For this review, take the finished solid that the model builds, in its own axes (mm). A direction names the side the tool comes from. Give positions to 0.01 mm unless a question says otherwise; leave off trailing zeros. Order: outer loops, then holes, each group sorted by start corner. A loop starts at its lowest first (then second) coordinate and runs counter-clockwise, first axis right, second up. Notation, with made-up numbers: M 8.25,86.25 L 35.25,86.25 A21 cw 35.25,98.25 Z; hole C -38.5,46.25 d1. An arc over 180 degrees is marked long. Use CSV: the item, a comma, the result in double quotes. Start each with the question number.
(1) Consider section D-D (x = 22.5). Write out the cut boundary in (y, z).
(2) Clearance check with flat-ended pins moving along their axes: P1, Ø9, axis at x = -1, z = -7.5, coming from the +Y side; P2, Ø1, axis at y = 4, z = 4.5, coming from the +X side; P3, Ø0.5, axis at x = 45.5, y = 3, coming from the +Z side; P4, Ø5, axis at x = 14.5, z = 2.5, coming from the +Y side. State where each tip first meets the part, or that it passes through.
(3) Consider section B-B (z = 33.5). Write out the cut boundary in (x, y).
(4) Tool access review of faces 1 (the face through (41.558, 2.768, 37.791)), 2 (the face through (-25.974, 3, 34)), 3 (the face through (-41.83, 0.99, -8.8)), 4 (the face through (-51, 2, 9.454)): name each direction out of +Z, -Z, +X, -X, +Y, -Y from which nothing blocks a thin tool from reaching the whole face with its end or side.
(5) Consider section A-A (x = 4). Write out the cut boundary in (y, z), and give its area (3 significant figures).
(6) Draft analysis for pull direction X (two halves, no side actions). For faces 5 (the face through (37, 4, 39)), 6 (the face through (14.226, 3, -3)), 7 (the face through (-42.463, 0.993, 41.416)), 8 (the face through (-48.627, 4, 15)), state which applies: pulls with the +X half, pulls with the -X half, needs draft (parallel to the pull), parting line crosses it, or undercut.
(7) Wall thickness on L1, parallel to Z at x = 2, y = 4.2; L2, parallel to X at y = 0.6, z = 41; L3, parallel to Z at x = -1, y = 1.1: over which ranges is each line inside the solid? List them lowest first. Write a range as from..to.
(8) Consider section C-C (z = 6.5). Write out the cut boundary in (x, y), and give its area (3 significant figures).
```python
from build123d import *

# Parameters (mm, degrees)
EXTRUDE_1_DEPTH     = 1.5
SKETCH_2_R          = 5
CUT_EXTRUDE_1_DEPTH = 0.5
SKETCH_11_R         = 2
SKETCH_11_W         = 12.230000074
SKETCH_11_H         = 11.974599949
EXTRUDE_5_DEPTH     = 2.539974634
SKETCH_13_R         = 2
SKETCH_13_W         = 4
SKETCH_13_H         = 10
TYPEC_2_DEPTH       = 5.7999746
LED_3_START         = -4.25
LED_3_DEPTH         = 2.75
LED_1_R             = 0.5
CUT_EXTRUDE_2_REACH = 75.864
SKETCH_15_R         = 2
EXTRUDE_START       = -4
SKETCH_16_R         = 4
SKETCH_16_R_2       = 1
EXTRUDE_4_DEPTH     = 2.5
LED_2_START         = -1.5
SKETCH_17_W         = 1
SKETCH_17_H         = 6
LED_2_DEPTH         = 0.5
SKETCH_18_W         = 40.2
SKETCH_18_H         = 3
EXTRUDE_2_DEPTH     = 3.5


with BuildPart() as part:
    # 草图1 → 凸台-拉伸1 (new body)
    with BuildSketch(Plane(origin=(0, 0, 0), x_dir=(1, 0, 0), z_dir=(0, 1, 0))):
        Polygon((-51.714401712, -9.454370264), (-55.976720775, -9.454370264), (-55.976720775, -21.428970213), (-51.714401712, -21.428970213), (-51.714401712, -47.841670238), (46.085598288, -47.841670238), (46.085598288, 16.958329762), (-51.714401712, 16.958329762), align=None)
    extrude(amount=EXTRUDE_1_DEPTH)

    # 草图2 → 防滑切除-拉伸1 (cut)
    with BuildSketch(Plane.XZ):
        with Locations(Location((-43.814401712, 39.941670238, 0), (0, 0, 270))):
            Circle(SKETCH_2_R)
        with Locations(Location((38.185598288, 39.941670238, 0), (0, 0, 90))):
            Circle(SKETCH_2_R)
        with Locations(Location((38.185598288, -9.058329762, 0), (0, 0, 90))):
            Circle(SKETCH_2_R)
        with Locations(Location((-43.814401712, -9.058329762, 0), (0, 0, 270))):
            Circle(SKETCH_2_R)
    extrude(amount=-CUT_EXTRUDE_1_DEPTH, mode=Mode.SUBTRACT)

    # 草图11 → 充电板档板凸台-拉伸5 (add)
    with BuildSketch(Plane.XZ):
        with Locations((-29.074401712, 29.928970213)):
            Circle(SKETCH_11_R)
        with Locations((-29.074401712, 0.954370264)):
            Circle(SKETCH_11_R)
        with Locations((-49.861720738, 15.441670239)):
            Rectangle(SKETCH_11_W, SKETCH_11_H)
    extrude(amount=-EXTRUDE_5_DEPTH)

    # 草图13 → TypeC支撑凸台-拉伸2 (add)
    with BuildSketch(Plane.XZ):
        with Locations(Location((-29.074401712, 29.928970213, 0), (0, 0, 90))):
            Circle(SKETCH_13_R)
        with Locations(Location((-29.074401712, 0.954370264, 0), (0, 0, 90))):
            Circle(SKETCH_13_R)
        with Locations((-46.626720701, 15.441670238)):
            Rectangle(SKETCH_13_W, SKETCH_13_H)
    extrude(amount=-TYPEC_2_DEPTH)

    # 草图14 → LED限位凸台-拉伸3 (add)
    with BuildSketch(Plane.XZ.offset(LED_3_START)):
        Polygon((45.085598288, 12.441670238), (45.085598288, 18.441670238), (46.085598288, 18.441670238), (46.085598288, 21.441670238), (42.085598288, 21.441670238), (42.085598288, 9.441670238), (46.085598288, 9.441670238), (46.085598288, 12.441670238), align=None)
    extrude(amount=LED_3_DEPTH)

    # LED限位圆角1
    led_1_edges = [part.edges().sort_by_distance(p)[0] for p in [
        (45.585598288, 4.25, 18.441670238),
        (45.585598288, 4.25, 12.441670238),
        (45.085598288, 4.25, 15.441670238),
        (-48.626720701, 5.7999746, 15.441670238),
    ]]
    fillet(led_1_edges, radius=LED_1_R)

    # 草图15 → 螺丝孔位切除-拉伸2 (cut, up to next)
    with BuildSketch(Plane.XZ, mode=Mode.PRIVATE) as cut_extrude_2_sk1:
        with Locations(Location((-43.814401712, -9.058329762, 0), (0, 0, 270))):
            Circle(SKETCH_15_R)
    cut_extrude_2_tool1 = extrude(cut_extrude_2_sk1.sketch, amount=-CUT_EXTRUDE_2_REACH, mode=Mode.PRIVATE) & part.part
    # 草图15 → 螺丝孔位切除-拉伸2 (cut, up to next)
    with BuildSketch(Plane.XZ, mode=Mode.PRIVATE) as cut_extrude_2_sk2:
        with Locations(Location((-43.814401712, 39.941670238, 0), (0, 0, 270))):
            Circle(SKETCH_15_R)
    cut_extrude_2_tool2 = extrude(cut_extrude_2_sk2.sketch, amount=-CUT_EXTRUDE_2_REACH, mode=Mode.PRIVATE) & part.part
    # 草图15 → 螺丝孔位切除-拉伸2 (cut, up to next)
    with BuildSketch(Plane.XZ, mode=Mode.PRIVATE) as cut_extrude_2_sk3:
        with Locations(Location((38.185598288, -9.058329762, 0), (0, 0, 270))):
            Circle(SKETCH_15_R)
    cut_extrude_2_tool3 = extrude(cut_extrude_2_sk3.sketch, amount=-CUT_EXTRUDE_2_REACH, mode=Mode.PRIVATE) & part.part
    # 草图15 → 螺丝孔位切除-拉伸2 (cut, up to next)
    with BuildSketch(Plane.XZ, mode=Mode.PRIVATE) as cut_extrude_2_sk4:
        with Locations(Location((38.185598288, 39.941670238, 0), (0, 0, 270))):
            Circle(SKETCH_15_R)
    cut_extrude_2_tool4 = extrude(cut_extrude_2_sk4.sketch, amount=-CUT_EXTRUDE_2_REACH, mode=Mode.PRIVATE) & part.part
    # 草图15 → 螺丝孔位切除-拉伸2 (cut, up to next)
    with BuildSketch(Plane.XZ, mode=Mode.PRIVATE) as cut_extrude_2_sk5:
        with Locations(Location((-2.814401712, 39.941670238, 0), (0, 0, 270))):
            Circle(SKETCH_15_R)
    cut_extrude_2_tool5 = extrude(cut_extrude_2_sk5.sketch, amount=-CUT_EXTRUDE_2_REACH, mode=Mode.PRIVATE) & part.part
    # 草图15 → 螺丝孔位切除-拉伸2 (cut, up to next)
    with BuildSketch(Plane.XZ, mode=Mode.PRIVATE) as cut_extrude_2_sk6:
        with Locations(Location((-2.814401712, -9.058329762, 0), (0, 0, 270))):
            Circle(SKETCH_15_R)
    cut_extrude_2_tool6 = extrude(cut_extrude_2_sk6.sketch, amount=-CUT_EXTRUDE_2_REACH, mode=Mode.PRIVATE) & part.part
    add(cut_extrude_2_tool1.solids().sort_by_distance((-43.814402, 0, -9.05833))[0], mode=Mode.SUBTRACT)
    add(cut_extrude_2_tool2.solids().sort_by_distance((-43.814402, 0, 39.94167))[0], mode=Mode.SUBTRACT)
    add(cut_extrude_2_tool3.solids().sort_by_distance((38.185598, 0, -9.05833))[0], mode=Mode.SUBTRACT)
    add(cut_extrude_2_tool4.solids().sort_by_distance((38.185598, 0, 39.94167))[0], mode=Mode.SUBTRACT)
    add(cut_extrude_2_tool5.solids().sort_by_distance((-2.814402, 0, 39.94167))[0], mode=Mode.SUBTRACT)
    add(cut_extrude_2_tool6.solids().sort_by_distance((-2.814402, 0, -9.05833))[0], mode=Mode.SUBTRACT)

    # 草图16 → 螺丝孔凸台-拉伸4 (add)
    # profile 1 of 6: a face of its own
    with BuildSketch(Plane.XZ.offset(EXTRUDE_START)):
        with Locations(Location((38.185598288, -9.058329762, 0), (0, 0, 270))):
            Circle(SKETCH_16_R)
        with Locations(Location((38.185598288, -9.058329762, 0), (0, 0, 270))):
            Circle(SKETCH_16_R_2, mode=Mode.SUBTRACT)
    # profile 2 of 6: a face of its own
    with BuildSketch(Plane.XZ.offset(EXTRUDE_START)):
        with Locations(Location((38.185598288, 39.941670238, 0), (0, 0, 270))):
            Circle(SKETCH_16_R)
        with Locations(Location((38.185598288, 39.941670238, 0), (0, 0, 270))):
            Circle(SKETCH_16_R_2, mode=Mode.SUBTRACT)
    # profile 3 of 6: a face of its own
    with BuildSketch(Plane.XZ.offset(EXTRUDE_START)):
        with Locations(Location((-43.814401712, -9.058329762, 0), (0, 0, 270))):
            Circle(SKETCH_16_R)
        with Locations(Location((-43.814401712, -9.058329762, 0), (0, 0, 270))):
            Circle(SKETCH_16_R_2, mode=Mode.SUBTRACT)
    # profile 4 of 6: a face of its own
    with BuildSketch(Plane.XZ.offset(EXTRUDE_START)):
        with Locations(Location((-43.814401712, 39.941670238, 0), (0, 0, 270))):
            Circle(SKETCH_16_R)
        with Locations(Location((-43.814401712, 39.941670238, 0), (0, 0, 270))):
            Circle(SKETCH_16_R_2, mode=Mode.SUBTRACT)
    # profile 5 of 6: a face of its own
    with BuildSketch(Plane.XZ.offset(EXTRUDE_START)):
        with Locations(Location((-2.814401712, 39.941670238, 0), (0, 0, 270))):
            Circle(SKETCH_16_R)
        with Locations(Location((-2.814401712, 39.941670238, 0), (0, 0, 270))):
            Circle(SKETCH_16_R_2, mode=Mode.SUBTRACT)
    # profile 6 of 6: a face of its own
    with BuildSketch(Plane.XZ.offset(EXTRUDE_START)):
        with Locations(Location((-2.814401712, -9.058329762, 0), (0, 0, 270))):
            Circle(SKETCH_16_R)
        with Locations(Location((-2.814401712, -9.058329762, 0), (0, 0, 270))):
            Circle(SKETCH_16_R_2, mode=Mode.SUBTRACT)
    extrude(amount=EXTRUDE_4_DEPTH)

    # 草图17 → LED灯嵌入切除-拉伸2 (cut)
    with BuildSketch(Plane.XZ.offset(LED_2_START)):
        with Locations((45.585598288, 15.441670238)):
            Rectangle(SKETCH_17_W, SKETCH_17_H)
    extrude(amount=LED_2_DEPTH, mode=Mode.SUBTRACT)

    # 草图18 → 散热板支撑凸台-拉伸2 (add)
    with BuildSketch(Plane(origin=(0, 1.5, 0), x_dir=(1, 0, 0), z_dir=(0, 1, 0))):
        with Locations((-5.874401712, 3.058329762)):
            Rectangle(SKETCH_18_W, SKETCH_18_H)
        with Locations((-5.874401712, -33.941670238)):
            Rectangle(SKETCH_18_W, SKETCH_18_H)
    extrude(amount=EXTRUDE_2_DEPTH)


solid = part.part
```
Check result:
1,outline,"M 0,-16.96 L 1.5,-16.96 L 1.5,47.84 L 0,47.84 Z"
2,P1,"stops at y = 5"
2,P2,"passes through"
2,P3,"stops at z = 21.44"
2,P4,"stops at y = 1.5"
3,outline,"M -51.71,0 L 46.09,0 L 46.09,1.5 L 14.23,1.5 L 14.23,5 L -25.97,5 L -25.97,1.5 L -51.71,1.5 Z"
4,face 1,"+Y"
4,face 2,"+Z, -Z, -X, +Y"
4,face 3,"-Y"
4,face 4,"-X, +Y"
5,outline,"M 0,-16.96 L 1.5,-16.96 L 1.5,-4.56 L 5,-4.56 L 5,-1.56 L 1.5,-1.56 L 1.5,32.44 L 5,32.44 L 5,35.44 L 1.5,35.44 L 1.5,47.84 L 0,47.84 Z"
5,area,"118 mm^2"
6,face 5,"needs draft"
6,face 6,"pulls with the +X half"
6,face 7,"undercut"
6,face 8,"pulls with the -X half"
7,L1,"z = -4.56..-1.56, 32.44..35.44"
7,L2,"x = -51.71..-45.51, -42.12..-4.51, -1.12..36.49, 39.88..46.09"
7,L3,"z = -16.96..-9.9, -8.22..39.1, 40.78..47.84"
8,outline,"M -51.71,0 L 46.09,0 L 46.09,1.5 L -51.71,1.5 Z"
8,area,"147 mm^2"
